from build123d import *

# Parameters (mm, degrees)
SKETCH1_W           = 63.5
SKETCH1_H           = 81.026
BOSS_EXTRUDE1_DEPTH = 4.826
SKETCH2_W           = 12.7
SKETCH2_H           = 4.826
CUT_EXTRUDE1_DEPTH  = 104.057037373
SKETCH3_W           = 4.826
SKETCH3_H           = 6.35
CUT_EXTRUDE2_DEPTH  = 4.826


with BuildPart() as part:
    # Sketch1 → Boss-Extrude1 (new body)
    with BuildSketch(Plane.XY):
        with Locations((31.75, 40.513)):
            Rectangle(SKETCH1_W, SKETCH1_H)
    extrude(amount=BOSS_EXTRUDE1_DEPTH)

    # Sketch2 → Cut-Extrude1 (cut, through all)
    with BuildSketch(Plane.XY.offset(4.826)):
        with Locations((6.35, 2.413)):
            Rectangle(SKETCH2_W, SKETCH2_H)
        with Locations((31.75, 2.413)):
            Rectangle(SKETCH2_W, SKETCH2_H)
        with Locations((57.15, 2.413)):
            Rectangle(SKETCH2_W, SKETCH2_H)
    extrude(amount=-CUT_EXTRUDE1_DEPTH, mode=Mode.SUBTRACT)

    # Sketch3 → Cut-Extrude2 (cut)
    with BuildSketch(Plane(origin=(0, 0, 0), x_dir=(-1, 0, 0), z_dir=(0, 0, -1))):
        with Locations((-50.927, 14.351)):
            Rectangle(SKETCH3_W, SKETCH3_H)
        with Locations((-12.573, 14.351)):
            Rectangle(SKETCH3_W, SKETCH3_H)
    extrude(amount=-CUT_EXTRUDE2_DEPTH, mode=Mode.SUBTRACT)


solid = part.part
Input: part model. Units: mm. Frame: model coordinates. A direction names the side the tool comes from. Coordinates: 2 decimals unless noted, no trailing zeros. Loops run counter-clockwise (first coordinate to the right, second up) from the corner with the lowest first, then second, coordinate; pieces in that order, holes last.
Q1. Material intervals for line 1 (Y direction, x = 12, z = 3.05); line 2 (Y direction, x = 49.5, z = 2.4); line 3 (X direction, y = 4, z = 0.7), sorted ascending.
Q2. Cut plane A-A (y = 16). Output: boundary loops of the cut face in (x, z).
Q3. Contact query for flat-ended pins moving along their axis: pin 1 (1.4 mm diameter, centred on y = 3, z = 1.5, fed in from -X); pin 2 (2.5 mm diameter, centred on y = 2, z = 2, fed in from +X). Output: stop coordinate, or through.
Q4. Set-up query: faces 1 (the face through (51, 17.526, 2)), 2 (the face through (57, 4.826, 2)), 3 (the face through (38.1, 2, 2)), 4 (the face through (6, 4.826, 2)). Return all of +Z, -Z, +X, -X, +Y, -Y with unobstructed straight access to the full face (end or side cutting, diameter ignored); none if empty.
Q5. Draft query along Y for faces 5 (the face through (19, 0, 2)), 6 (the face through (13, 11.176, 2)), 7 (the face through (31, 81.026, 2)), 8 (the face through (25.4, 2, 2)). Return one class per face: +Y half, -Y half, draft (parallel to the pull), parting line (faces both ways), or undercut.
Q6. Cut plane B-B (z = 1.2). Output: boundary loops of the cut face in (x, y), then the cut area to 3 significant figures.
Q7. Cut plane C-C (x = 6). Output: boundary loops of the cut face in (y, z), then the cut area to 3 significant figures.
Working result:
1. line 1: y = 4.83 to 11.18, 17.53 to 81.03
1. line 2: y = 0 to 11.18, 17.53 to 81.03
1. line 3: x = 12.7 to 25.4, 38.1 to 50.8
2. outline: (0, 0) - (10.16, 0) - (10.16, 4.83) - (0, 4.83) - close; (14.99, 0) - (48.51, 0) - (48.51, 4.83) - (14.99, 4.83) - close; (53.34, 0) - (63.5, 0) - (63.5, 4.83) - (53.34, 4.83) - close
3. pin 1: stops at x = 12.7
3. pin 2: stops at x = 50.8
4. face 1: +Z, -Z
4. face 2: +Z, -Z, +X, -Y
4. face 3: +Z, -Z, -Y
4. face 4: +Z, -Z, -X, -Y
5. face 5: -Y half
5. face 6: undercut
5. face 7: +Y half
5. face 8: draft
6. outline: (0, 4.83) - (12.7, 4.83) - (12.7, 0) - (25.4, 0) - (25.4, 4.83) - (38.1, 4.83) - (38.1, 0) - (50.8, 0) - (50.8, 4.83) - (63.5, 4.83) - (63.5, 81.03) - (0, 81.03) - close; hole (10.16, 11.18) - (14.99, 11.18) - (14.99, 17.53) - (10.16, 17.53) - close; hole (48.51, 11.18) - (53.34, 11.18) - (53.34, 17.53) - (48.51, 17.53) - close
6. area: 4,900 mm2
7. outline: (4.83, 0) - (81.03, 0) - (81.03, 4.83) - (4.83, 4.83) - close
7. area: 368 mm2
